Could you check a few things on this model? Use its own coordinates, in mm. A direction names the side the tool comes from. Coordinates: 2 decimals unless noted, no trailing zeros. Order: outer loops, then holes, each group sorted by start corner. A loop starts at its lowest first (then second) coordinate and runs counter-clockwise, first axis right, second up. Notation, with made-up numbers: (20, 72) -> (69, 72) arc R13 ccw to (69, 76) -> close; hole circle Ø4 at (-2.5, 44). An arc over 180 degrees is marked (long way). Use a Markdown table: item, result. Add a question column.
1) If I drill on L1, parallel to Z at x = 5, y = -10; L2, parallel to X at y = -17, z = 31; L3, parallel to Z at x = 66.5, y = -47, over which ranges is the centre line in solid material (lowest first)? Write a range as [from, to].
2) Which directions (+Z, -Z, +X, -X, +Y, -Y) give clear straight access to the entire face, cutting with the end or side of a thin tool? Please do faces 4 (the flat face through (65, -10, 236)), 5 (the flat face through (65, -10, 90)), 6 (the flat face through (65, -45, 82)), 7 (the flat face through (39, -67.5, 147)), 8 (the flat face through (40, -50, 212)).
3) If we section it at B-B (z = 143.5): Write out the boundary of the cut face in (x, y).
4) If we section it at A-A (z = 45): Write out the boundary of the cut face in (x, y).
5) Thinking about a two-plate mould opening in Y: for faces 1 (the flat face through (40, -46, 222.5)), 2 (the flat face through (36.904, -95.695, -21.144)), 3 (the cylindrical face through (72, -10, 48)), which applies, +Y half, -Y half, draft (parallel to the pull), parting line (faces both ways), or undercut?
6) Will these pins go through, and if not, where does the flat tip stop? pin 1 Ø5 at (y, z) = (-10, 45) entering from -X; pin 2 Ø4 at (x, z) = (34.5, 238.5) entering from -Y; pin 3 Ø10 at (y, z) = (-13, 223.5) entering from +X; pin 4 Ø10 at (x, y) = (38, -43.5) entering from -Z.
7) If we section it at C-C (y = -55): Give the number of separate pieces and of enclosed holes in the cut face, plus the area to 3 significant figures.
8) If we section it at D-D (z = 228.5): Write out the boundary of the cut face in (x, y), plus the area to 3 significant figures.
```python
from build123d import *
from build123d.topology import SkipClean

# Parameters (mm, degrees)
SKETCH_1_R               = 3
SKETCH_1_R_2             = 2
EXTRUDE_1_DEPTH          = 80
CUT_EXTRUDE_4_REACH      = 297.59
CUT_EXTRUDE_4_END_RADIUS = 55
SKETCH_4_W               = 15
SKETCH_4_H               = 20
SKETCH_5_W               = 75
SKETCH_5_H               = 45
EXTRUDE_2_DEPTH          = 22.15
SKETCH_10_R              = 12.5
CUT_EXTRUDE_5_DEPTH      = 60
SKETCH_12_R              = 3
SKETCH_12_R_2            = 1.5
CUT_EXTRUDE_6_DEPTH      = 15
FILLET_1_R               = 10
SKETCH_13_W              = 50
SKETCH_13_H              = 20
CUT_EXTRUDE_7_DEPTH      = 280.131397208
CUT_EXTRUDE_8_REACH      = 303.476
CUT_EXTRUDE_8_END_RADIUS = 55
SKETCH_14_W              = 15
SKETCH_14_H              = 20
SKETCH_15_W              = 50
SKETCH_15_H              = 10
EXTRUDE_3_DEPTH          = 20


with BuildPart() as part:
    # Эскиз1 → Бобышка-Вытянуть1 (new body)
    with BuildSketch(Plane(origin=(0, 0, 0), x_dir=(0, 0, -1), z_dir=(1, 0, 0))):
        with BuildLine():
            Line((0, 0), (0, -95))
            Line((0, -95), (-27.5, -95))
            ThreePointArc((-27.5, -95), (-40.221163687, -59.821881801), (-72.5, -40.916730868))
            Line((-72.5, -40.916730868), (-72.5, -50))
            Line((-72.5, -50), (-92.5, -50))
            Line((-92.5, -50), (-92.5, -40.916730868))
            ThreePointArc((-92.5, -40.916730868), (-114.23345294, -50.077979069), (-130.131397208, -67.5))
            Line((-130.131397208, -67.5), (-164.868602792, -67.5))
            ThreePointArc((-164.868602792, -67.5), (-180.76654706, -50.077979069), (-202.5, -40.916730868))
            Line((-202.5, -40.916730868), (-202.5, -50))
            Line((-202.5, -50), (-222.5, -50))
            Line((-222.5, -50), (-222.5, -40.916730868))
            ThreePointArc((-222.5, -40.916730868), (-244.23345294, -50.077979069), (-260.131397208, -67.5))
            Line((-260.131397208, -67.5), (-280.131397208, -67.5))
            Line((-280.131397208, -67.5), (-280.131397208, 0))
            Line((-280.131397208, 0), (0, 0))
        make_face()
        with Locations((-45, -10)):
            Circle(SKETCH_1_R, mode=Mode.SUBTRACT)
        with Locations((-122.5, -10)):
            Circle(SKETCH_1_R, mode=Mode.SUBTRACT)
        with Locations((-270.131397208, -10)):
            Circle(SKETCH_1_R_2, mode=Mode.SUBTRACT)
        with Locations((-260.131397208, -10)):
            Circle(SKETCH_1_R_2, mode=Mode.SUBTRACT)
    extrude(amount=EXTRUDE_1_DEPTH)

    # Вырез-Вытянуть4: up to this cylinder (the profile starts inside it)
    with SkipClean():  # the faces are left unmerged after this step: merging them gives an invalid solid
        cut_extrude_4_end = Plane(origin=(40, -95, 82.5), z_dir=(-1, 0, 0)) * Cylinder(CUT_EXTRUDE_4_END_RADIUS, 771.18, mode=Mode.PRIVATE)
        # Эскиз4 → Вырез-Вытянуть4 (cut, up to the surface)
        with BuildSketch(Plane.XZ.offset(50), mode=Mode.PRIVATE) as cut_extrude_4_sk1:
            with Locations((7.5, 82.5)):
                Rectangle(SKETCH_4_W, SKETCH_4_H)
        cut_extrude_4_tool1 = extrude(cut_extrude_4_sk1.sketch, amount=-CUT_EXTRUDE_4_REACH, mode=Mode.PRIVATE) & cut_extrude_4_end
        add(cut_extrude_4_tool1.solids().sort_by_distance((7.5, -50, 82.5))[0], mode=Mode.SUBTRACT)
        # Эскиз4 → Вырез-Вытянуть4 (cut, up to the surface)
        with BuildSketch(Plane.XZ.offset(50), mode=Mode.PRIVATE) as cut_extrude_4_sk2:
            with Locations((72.5, 82.5)):
                Rectangle(SKETCH_4_W, SKETCH_4_H)
        cut_extrude_4_tool2 = extrude(cut_extrude_4_sk2.sketch, amount=-CUT_EXTRUDE_4_REACH, mode=Mode.PRIVATE) & cut_extrude_4_end
        add(cut_extrude_4_tool2.solids().sort_by_distance((72.5, -50, 82.5))[0], mode=Mode.SUBTRACT)

    # Эскиз5 → Бобышка-Вытянуть2 (add, symmetric)
    with SkipClean():  # the faces are left unmerged after this step: merging them gives an invalid solid
        with BuildSketch(Plane(origin=(-21.13620668, -36.608983849, 0), x_dir=(-0.8660254037844379, 0.5000000000000012, 0), z_dir=(0.5000000000000012, 0.8660254037844379, 0))):
            with Locations((-79.282032303, -22.5)):
                Rectangle(SKETCH_5_W, SKETCH_5_H)
        extrude(amount=EXTRUDE_2_DEPTH, both=True)

    # Эскиз10 → Вырез-Вытянуть5 (cut)
    with SkipClean():  # the faces are left unmerged after this step: merging them gives an invalid solid
        with BuildSketch(Plane(origin=(36.184301396, -20.891016151, 0), x_dir=(0, 0, 1), z_dir=(-0.866025403784438, 0.5000000000000012, 0))):
            with Locations(Location((-22.5, -42.27241336, 0), (0, 0, 270))):
                Circle(SKETCH_10_R)
        extrude(amount=-CUT_EXTRUDE_5_DEPTH, mode=Mode.SUBTRACT)

    # Эскиз12 → Вырез-Вытянуть6 (cut)
    with SkipClean():  # the faces are left unmerged after this step: merging them gives an invalid solid
        with BuildSketch(Plane(origin=(88.145825623, -50.891016151, 0), x_dir=(0, 0, 1), z_dir=(-0.866025403784438, 0.5000000000000012, 0))):
            with Locations(Location((-22.5, -42.27241336, 0), (0, 0, 270))):
                Circle(SKETCH_12_R)
            with Locations(Location((-22.5, -33.77241336, 0), (0, 0, 270))):
                Circle(SKETCH_12_R_2)
            with Locations(Location((-14, -42.27241336, 0), (0, 0, 270))):
                Circle(SKETCH_12_R_2)
            with Locations(Location((-22.5, -50.77241336, 0), (0, 0, 270))):
                Circle(SKETCH_12_R_2)
            with Locations(Location((-31, -42.27241336, 0), (0, 0, 270))):
                Circle(SKETCH_12_R_2)
        extrude(amount=-CUT_EXTRUDE_6_DEPTH, mode=Mode.SUBTRACT)

    # Скругление1
    fillet_1_edges = [part.edges().sort_by_distance(p)[0] for p in [
        (52.3125, -104.591231347, 0),
        (36.449047358, -95.432462694, -45),
        (58.599047358, -57.067537306, -45),
        (85.5375, -72.620460191, 0),
    ]]
    fillet(fillet_1_edges, radius=FILLET_1_R)

    # Эскиз13 → Вырез-Вытянуть7 (cut)
    with BuildSketch(Plane(origin=(0, 0, 0), x_dir=(-1, 0, 0), z_dir=(0, 0, -1))):
        with Locations((-40, -10)):
            Rectangle(SKETCH_13_W, SKETCH_13_H)
    extrude(amount=-CUT_EXTRUDE_7_DEPTH, mode=Mode.SUBTRACT)

    # Вырез-Вытянуть8: up to this cylinder (the profile starts inside it)
    with SkipClean():  # the faces are left unmerged after this step: merging them gives an invalid solid
        cut_extrude_8_end = Plane(origin=(40, -95, 212.5), z_dir=(-1, 0, 0)) * Cylinder(CUT_EXTRUDE_8_END_RADIUS, 782.952, mode=Mode.PRIVATE)
        # Эскиз14 → Вырез-Вытянуть8 (cut, up to the surface)
        with BuildSketch(Plane.XZ.offset(50), mode=Mode.PRIVATE) as cut_extrude_8_sk1:
            with Locations((7.5, 212.5)):
                Rectangle(SKETCH_14_W, SKETCH_14_H)
        cut_extrude_8_tool1 = extrude(cut_extrude_8_sk1.sketch, amount=-CUT_EXTRUDE_8_REACH, mode=Mode.PRIVATE) & cut_extrude_8_end
        add(cut_extrude_8_tool1.solids().sort_by_distance((7.5, -50, 212.5))[0], mode=Mode.SUBTRACT)
        # Эскиз14 → Вырез-Вытянуть8 (cut, up to the surface)
        with BuildSketch(Plane.XZ.offset(50), mode=Mode.PRIVATE) as cut_extrude_8_sk2:
            with Locations((72.5, 212.5)):
                Rectangle(SKETCH_14_W, SKETCH_14_H)
        cut_extrude_8_tool2 = extrude(cut_extrude_8_sk2.sketch, amount=-CUT_EXTRUDE_8_REACH, mode=Mode.PRIVATE) & cut_extrude_8_end
        add(cut_extrude_8_tool2.solids().sort_by_distance((72.5, -50, 212.5))[0], mode=Mode.SUBTRACT)

    # Эскиз15 → Бобышка-Вытянуть3 (add)
    with SkipClean():  # the faces are left unmerged after this step: merging them gives an invalid solid
        with BuildSketch(Plane(origin=(0, -20, 0), x_dir=(1, 0, 0), z_dir=(0, 1, 0))):
            with Locations((40, -187.5)):
                Rectangle(SKETCH_15_W, SKETCH_15_H)
        extrude(amount=EXTRUDE_3_DEPTH)


solid = part.part
```
Answer sheet:
| question | item | result |
|---|---|---|
| 1 | L1 | [0, 42], [48, 119.5], [125.5, 258.13], [262.13, 268.13], [272.13, 280.13] |
| 1 | L2 | [0, 15], [65, 80] |
| 1 | L3 | [0, 55.65], [109.35, 185.65], [239.35, 280.13] |
| 2 | face 4 | +Z, +Y |
| 2 | face 5 | -Z, +Y |
| 2 | face 6 | +X, -Y |
| 2 | face 7 | +Z, +X, -X, -Y |
| 2 | face 8 | +X, -X, -Y |
| 3 | outline | (0, -67.5) -> (80, -67.5) -> (80, 0) -> (65, 0) -> (65, -20) -> (15, -20) -> (15, 0) -> (0, 0) -> close |
| 4 | outline | (0, -54.77) -> (80, -54.77) -> (80, -13) -> (65, -13) -> (65, -20) -> (15, -20) -> (15, -13) -> (0, -13) -> close; (0, -7) -> (15, -7) -> (15, 0) -> (0, 0) -> close; (65, -7) -> (80, -7) -> (80, 0) -> (65, 0) -> close |
| 5 | face 1 | draft |
| 5 | face 2 | -Y half |
| 5 | face 3 | undercut |
| 6 | pin 1 | through |
| 6 | pin 2 | y = -47.66 |
| 6 | pin 3 | x = 80 |
| 6 | pin 4 | z = -42.64 |
| 7 | separate pieces | 3 |
| 7 | enclosed holes | 0 |
| 7 | area | 11,700 mm2 |
| 8 | outline | (0, -42.38) -> (80, -42.38) -> (80, 0) -> (65, 0) -> (65, -20) -> (15, -20) -> (15, 0) -> (0, 0) -> close |
| 8 | area | 2,390 mm2 |
